```python
from build123d import *
from build123d.topology import SkipClean

# Parameters (mm, degrees)
SKETCH2_W           = 240
SKETCH2_H           = 68
BOSS_EXTRUDE1_DEPTH = 15
SKETCH4_R           = 25
SKETCH4_R_2         = 15
BOSS_EXTRUDE4_DEPTH = 40
CUT_EXTRUDE2_START  = -40
SKETCH7_R           = 15
CUT_EXTRUDE2_DEPTH  = 40
BOSS_EXTRUDE5_DEPTH = 30
CUT_EXTRUDE3_DEPTH  = 77
RIB3_REACH          = 138.312
SKETCH11_WALL_W     = 307.624283584
SKETCH11_WALL_H     = 10
BOSS_EXTRUDE6_DEPTH = 8
SKETCH13_R          = 18
BOSS_EXTRUDE7_DEPTH = 42
SKETCH14_R          = 10
CUT_EXTRUDE4_DEPTH  = 67


with BuildPart() as part:
    # Sketch2 → Boss-Extrude1 (new body)
    with BuildSketch(Plane(origin=(0, 0, 0), x_dir=(1, 0, 0), z_dir=(0, 1, 0))):
        Rectangle(SKETCH2_W, SKETCH2_H)
    extrude(amount=BOSS_EXTRUDE1_DEPTH)

    # Sketch4 → Boss-Extrude4 (add)
    with BuildSketch(Plane(origin=(0, 15, 0), x_dir=(1, 0, 0), z_dir=(0, 1, 0))):
        with Locations(Location((-82, 0, 0), (0, 0, 270))):
            Circle(SKETCH4_R)
        with Locations(Location((-82, 0, 0), (0, 0, 270))):
            Circle(SKETCH4_R_2, mode=Mode.SUBTRACT)
    extrude(amount=BOSS_EXTRUDE4_DEPTH)

    # Sketch7 → Cut-Extrude2 (cut)
    with BuildSketch(Plane(origin=(0, 15, 0), x_dir=(1, 0, 0), z_dir=(0, 1, 0)).offset(CUT_EXTRUDE2_START)):
        with Locations(Location((-82, 0, 0), (0, 0, 270))):
            Circle(SKETCH7_R)
    extrude(amount=CUT_EXTRUDE2_DEPTH, mode=Mode.SUBTRACT)

    # Sketch8 → Boss-Extrude5 (add)
    with BuildSketch(Plane(origin=(0, 15, 0), x_dir=(1, 0, 0), z_dir=(0, 1, 0))):
        with BuildLine():
            Line((-4, 20), (26, 20))
            ThreePointArc((26, 20), (46, 0), (26, -20))
            Line((26, -20), (-4, -20))
            ThreePointArc((-4, -20), (-24, 0), (-4, 20))
        make_face()
    extrude(amount=BOSS_EXTRUDE5_DEPTH)

    # Sketch9 → Cut-Extrude3 (cut)
    with BuildSketch(Plane(origin=(0, 45, 0), x_dir=(1, 0, 0), z_dir=(0, 1, 0))):
        with BuildLine():
            Line((-4, -10), (26, -10))
            ThreePointArc((26, -10), (36, 0), (26, 10))
            Line((26, 10), (-4, 10))
            ThreePointArc((-4, 10), (-14, 0), (-4, -10))
        make_face()
    extrude(amount=-CUT_EXTRUDE3_DEPTH, mode=Mode.SUBTRACT)

    # Sketch11 wall → Rib3 (add, up to next)
    with BuildSketch(Plane(origin=(-40.5, 35, 0), x_dir=(1, 0, 0), z_dir=(0, 1, 0)), mode=Mode.PRIVATE) as rib3_sk1:
        Rectangle(SKETCH11_WALL_W, SKETCH11_WALL_H)
    rib3_tool1 = extrude(rib3_sk1.sketch, amount=-RIB3_REACH, mode=Mode.PRIVATE) - part.part
    add(rib3_tool1.solids().sort_by_distance((-40.5, 35, 0))[0])

    # Sketch12 → Boss-Extrude6 (add)
    with BuildSketch(Plane(origin=(120, 0, 0), x_dir=(0, 0, -1), z_dir=(1, 0, 0))):
        with BuildLine():
            Line((-18, 95), (-34, 15))
            Line((-34, 15), (34, 15))
            Line((34, 15), (18, 95))
            ThreePointArc((18, 95), (0, 113), (-18, 95))
        make_face()
    extrude(amount=-BOSS_EXTRUDE6_DEPTH)

    # Sketch13 → Boss-Extrude7 (add)
    with SkipClean():  # the faces are left unmerged after this step: merging them gives an invalid solid
        with BuildSketch(Plane.ZY.offset(-112)):
            with Locations((0, 95)):
                Circle(SKETCH13_R)
        extrude(amount=BOSS_EXTRUDE7_DEPTH)
    add(part.part.scale(1), mode=Mode.REPLACE)  # the faces are merged on a copy

    # Sketch14 → Cut-Extrude4 (cut)
    with BuildSketch(Plane.ZY.offset(-70)):
        with Locations((0, 95)):
            Circle(SKETCH14_R)
    extrude(amount=-CUT_EXTRUDE4_DEPTH, mode=Mode.SUBTRACT)


solid = part.part
```
Work out the finished part from the listing and answer in its coordinate system (mm). A direction names the side the tool comes from. Round coordinates to 2 decimals unless told otherwise and drop trailing zeros. Loops run counter-clockwise (first coordinate to the right, second up) from the corner with the lowest first, then second, coordinate; pieces in that order, holes last.
(1) The part is cut by section D-D, the plane y = 91. Give the vertices of the cut face in (x, z), and give its area (3 significant figures).
Computed values:
outline: (70, -17.55) - (112, -17.55) - (112, -18.8) - (120, -18.8) - (120, -9.17) - (70, -9.17) - close; (70, 9.17) - (120, 9.17) - (120, 18.8) - (112, 18.8) - (112, 17.55) - (70, 17.55) - close
area: 858 mm2
(2) The part is cut by section C-C, the plane z = 0. Give the vertices of the cut face in (x, y).
Computed values:
outline: (-120, 0) - (-97, 0) - (-97, 55) - (-107, 55) - (-107, 15) - (-120, 15) - close; (-67, 0) - (-14, 0) - (-14, 45) - (-24, 45) - (-24, 35) - (-57, 35) - (-57, 55) - (-67, 55) - close; (36, 0) - (120, 0) - (120, 85) - (70, 85) - (70, 77) - (112, 77) - (112, 15) - (46, 15) - (46, 45) - (36, 45) - close; (70, 105) - (120, 105) - (120, 113) - (70, 113) - close
(3) For faces 5 (the cylindrical face through (46, 30, 0)), 6 (the flat face through (70, 87, 8)), 7 (the flat face through (11, 30, 20)), determine the directions among +Z, -Z, +X, -X, +Y, -Y from which every point of the face is accessible in a straight line to the end or side of a thin tool.
Computed values:
face 5: +Y
face 6: +Z, -Z, -X, +Y
face 7: +Z, +Y
(4) Find the intervals of material crossed by L1, parallel to X at y = 44.5, z = -0.5 (1 decimal); L2, parallel to Y at x = 81, z = 0; L3, parallel to X at y = 18.5, z = 0, in increasing order.
Computed values:
L1: x = -107 to -97, -67 to -57, -24 to -14, 36 to 46, 112 to 120
L2: y = 0 to 15, 77 to 85, 105 to 113
L3: x = -107 to -97, -67 to -14, 36 to 46, 112 to 120
(5) The part is cut by section B-B, the plane x = -82. Give the vertices of the cut face in (y, z), and give its area (3 significant figures).
Computed values:
outline: (0, -34) - (15, -34) - (15, -25) - (55, -25) - (55, -15) - (0, -15) - close; (0, 15) - (55, 15) - (55, 25) - (15, 25) - (15, 34) - (0, 34) - close
area: 1,370 mm2
(6) The mould has two halves that part along Y. Classify faces 1 (the flat face through (116.06, 54.44, -26.11)), 2 (the flat face through (-41, 25, -5)), 3 (the flat face through (-6, 15, -23)), 4 (the flat face through (112, 47, 0)): pulls with the +Y half, pulls with the -Y half, needs draft (parallel to the pull), parting line crosses it, or undercut.
Computed values:
face 1: pulls with the +Y half
face 2: needs draft
face 3: undercut
face 4: undercut
(7) Each of these flat-tipped pins is pushed along its axis until it touches: P1, Ø3, axis at y = 36, z = -13, coming from the -X side; P2, Ø2, axis at x = 83.5, z = 1.5, coming from the +Y side; P3, Ø6, axis at x = 68, y = 82.5, coming from the +Z side. Where does it stop, or does it pass through?
Computed values:
P1: stops at x = -104.2
P2: stops at y = 112.99
P3: stops at z = 14.79
(8) The part is cut by section A-A, the plane y = 27. Give the vertices of the cut face in (x, z).
Computed values:
outline: (-57.51, -5) - (-23.36, -5) arc R20 ccw to (-4, -20) - (26, -20) arc R20 ccw to (26, 20) - (-4, 20) arc R20 ccw to (-23.36, 5) - (-57.51, 5) arc R25 ccw (long way) to start; (112, -31.6) - (120, -31.6) - (120, 31.6) - (112, 31.6) - close; hole circle Ø30 at (-82, 0); hole (-4, -10) - (26, -10) arc R10 ccw to (26, 10) - (-4, 10) arc R10 ccw to start
